Can you work these out from the model? Positions are in its coordinate system, mm. A direction names the side the tool comes from. Give positions to 0.01 mm unless a question says otherwise; leave off trailing zeros. Write each loop counter-clockwise with the first axis right and the second up, starting at its lowest first coordinate (ties: lowest second). Pieces come first, ordered by that corner, then holes. Notation, with made-up numbers: (70.25, -8.5) -> (122.25, -8.5) arc R12 ccw to (122.25, 12.5) -> close; hole circle Ø6 at (43, 44). An arc over 180 degrees is marked (long way). One line per item, written item: value.
from build123d import *

# Parameters (mm, degrees)
SKETCH1_W           = 15
SKETCH1_H           = 304.8
BOSS_EXTRUDE1_DEPTH = 5.588
SKETCH2_R           = 1.75
CUT_EXTRUDE1_DEPTH  = 217.796734309
SKETCH3_R           = 1.75
CUT_EXTRUDE2_DEPTH  = 217.796734309
FILLET1_R           = 6


with BuildPart() as part:
    # Sketch1 → Boss-Extrude1 (new body)
    with BuildSketch(Plane.XY):
        with Locations((2.310829902, -64.102530885)):
            Rectangle(SKETCH1_W, SKETCH1_H)
    extrude(amount=BOSS_EXTRUDE1_DEPTH)

    # Sketch2 → Cut-Extrude1 (cut, through all)
    with BuildSketch(Plane.XY.offset(5.588)):
        with Locations((2.310829902, 78.297469115)):
            Circle(SKETCH2_R)
        with Locations((2.310829902, 58.297469115)):
            Circle(SKETCH2_R)
        with Locations((2.310829902, 50.297469115)):
            Circle(SKETCH2_R)
        with Locations((2.310829902, 42.297469115)):
            Circle(SKETCH2_R)
        with Locations((2.310829902, 34.297469115)):
            Circle(SKETCH2_R)
        with Locations((2.310829902, 26.297469115)):
            Circle(SKETCH2_R)
        with Locations((2.310829902, -50.762845209)):
            Circle(SKETCH2_R)
        with Locations((2.310829902, -96.702530885)):
            Circle(SKETCH2_R)
        with BuildLine():
            Line((0.029482749, -1.702530885), (4.592177054, -1.702530885))
            ThreePointArc((4.592177054, -1.702530885), (6.006390617, -2.288317323), (6.592177054, -3.702530885))
            Line((6.592177054, -3.702530885), (6.592177054, -39.702530885))
            ThreePointArc((6.592177054, -39.702530885), (6.006390617, -41.116744448), (4.592177054, -41.702530885))
            Line((4.592177054, -41.702530885), (0.029482749, -41.702530885))
            ThreePointArc((0.029482749, -41.702530885), (-1.384730813, -41.116744448), (-1.970517251, -39.702530885))
            Line((-1.970517251, -39.702530885), (-1.970517251, -3.702530885))
            ThreePointArc((-1.970517251, -3.702530885), (-1.384730813, -2.288317323), (0.029482749, -1.702530885))
        make_face()
        with BuildLine():
            Line((0.029482749, -61.702530885), (4.592177054, -61.702530885))
            ThreePointArc((4.592177054, -61.702530885), (6.006390617, -62.288317323), (6.592177054, -63.702530885))
            Line((6.592177054, -63.702530885), (6.592177054, -89.702530885))
            ThreePointArc((6.592177054, -89.702530885), (6.006390617, -91.116744448), (4.592177054, -91.702530885))
            Line((4.592177054, -91.702530885), (0.029482749, -91.702530885))
            ThreePointArc((0.029482749, -91.702530885), (-1.384730813, -91.116744448), (-1.970517251, -89.702530885))
            Line((-1.970517251, -89.702530885), (-1.970517251, -63.702530885))
            ThreePointArc((-1.970517251, -63.702530885), (-1.384730813, -62.288317323), (0.029482749, -61.702530885))
        make_face()
    extrude(amount=-CUT_EXTRUDE1_DEPTH, mode=Mode.SUBTRACT)

    # Sketch3 → Cut-Extrude2 (cut, through all)
    with BuildSketch(Plane.XY.offset(5.588)):
        with Locations((2.310829902, -208.502530885)):
            Circle(SKETCH3_R)
    extrude(amount=-CUT_EXTRUDE2_DEPTH, mode=Mode.SUBTRACT)

    # Fillet1
    fillet1_edges = [part.edges().sort_by_distance(p)[0] for p in [
        (9.810829902, -216.502530885, 2.794),
        (-5.189170098, -216.502530885, 2.794),
    ]]
    fillet(fillet1_edges, radius=FILLET1_R)


solid = part.part
1) Will these pins go through, and if not, where does the flat tip stop? pin 1 (4.5 mm diameter, centred on x = 2.31, y = 34.3, fed in from -Z); pin 2 (3 mm diameter, centred on x = 2.31, y = -96.7, fed in from +Z); pin 3 (1 mm diameter, centred on x = -3, z = 4, fed in from -Y); pin 4 (1.5 mm diameter, centred on x = -1.5, z = 1, fed in from -Y).
Answer list:
pin 1: stops at z = 0
pin 2: passes through
pin 3: stops at y = -215.51
pin 4: stops at y = -216.3
2) For faces 1 (the face through (-1.971, -22, 3)), 2 (the face through (-3, -62, 5.588)), which set-ups out of +Z, -Z, +X, -X, +Y, -Y let a thin tool reach every point of the face, with its end or its side?
Answer list:
face 1: +Z, -Z
face 2: +Z, +X, -X, +Y, -Y
3) If we section it at A-A (y = -15): Write out the boundary of the cut face in (x, z).
Answer list:
outline: (-5.19, 0) -> (-1.97, 0) -> (-1.97, 5.59) -> (-5.19, 5.59) -> close; (6.59, 0) -> (9.81, 0) -> (9.81, 5.59) -> (6.59, 5.59) -> close
4) If we section it at B-B (z = 3.15): State how many separate pieces and enclosed holes the cut face has, and give its area (3 significant figures).
Answer list:
separate pieces: 1
enclosed holes: 11
area: 3,880 mm^2
5) We'd pull the mould along Y, two halves only. Please class faces 3 (the face through (8, -214.8, 2.8)), 4 (the face through (9.811, -63, 3)), 5 (the face through (6.592, -21, 3)), 6 (the face through (2, 88.297, 3)): released by +Y, released by -Y, zero draft, split by the parting line, or undercut.
Answer list:
face 3: released by -Y
face 4: zero draft
face 5: undercut
face 6: released by +Y
6) I need wall thicknesses on L1, parallel to Y at x = 4.25, z = 0.7; L2, parallel to Y at x = 4.75, z = 4.15; L3, parallel to X at y = -37.5, z = 5.35. Which ranges of each line are inside material? Lowest first, please.
Answer list:
L1: y = -216.49 to -91.7, -61.7 to -41.7, -1.7 to 88.3
L2: y = -216.43 to -91.7, -61.71 to -41.7, -1.71 to 88.3
L3: x = -5.19 to -1.97, 6.59 to 9.81
